```python
from build123d import *

# Parameters (mm, degrees)
F0_W     = 120
F0_H     = 60
F1_DEPTH = 3
F3_DEPTH = 1
F5_DEPTH = 1
F6_D     = 3.3
F7_D     = 3.3


with BuildPart() as f1:
    # F0 (on Top) → F1 (new body)
    with BuildSketch(Plane.XY):
        with Locations((63.9999989198, 30)):
            Rectangle(F0_W, F0_H)
    extrude(amount=F1_DEPTH)

    # F2 (on face) → F3 (cut)
    with BuildSketch(Plane.XY.offset(3)):
        with BuildLine():
            ThreePointArc((14.6999989198, 54.4), (13.2062435039, 58.0062445841), (9.5999989198, 59.5))
            Line((9.5999989198, 59.5), (9.5999989198, 54.4))
            Line((9.5999989198, 54.4), (14.6999989198, 54.4))
        make_face()
        with BuildLine():
            Line((9.5999989198, 49.3), (9.5999989198, 54.4))
            Line((9.5999989198, 54.4), (4.4999989198, 54.4))
            ThreePointArc((4.4999989198, 54.4), (5.9937543357, 50.7937554159), (9.5999989198, 49.3))
        make_face()
        with BuildLine():
            Line((14.6999989198, 54.4), (9.5999989198, 54.4))
            Line((9.5999989198, 54.4), (9.5999989198, 49.3))
            ThreePointArc((9.5999989198, 49.3), (13.2062435039, 50.7937554159), (14.6999989198, 54.4))
        make_face()
        with BuildLine():
            Line((9.5999989198, 5.6), (9.5999989198, 10.7))
            ThreePointArc((9.5999989198, 10.7), (5.9937543357, 9.2062445841), (4.4999989198, 5.6))
            Line((4.4999989198, 5.6), (9.5999989198, 5.6))
        make_face()
        with BuildLine():
            ThreePointArc((14.6999989198, 5.6), (13.2062435039, 9.2062445841), (9.5999989198, 10.7))
            Line((9.5999989198, 10.7), (9.5999989198, 5.6))
            Line((9.5999989198, 5.6), (14.6999989198, 5.6))
        make_face()
        with BuildLine():
            Line((9.5999989198, 5.6), (4.4999989198, 5.6))
            ThreePointArc((4.4999989198, 5.6), (5.9937543357, 1.9937554159), (9.5999989198, 0.5))
            Line((9.5999989198, 0.5), (9.5999989198, 5.6))
        make_face()
        with BuildLine():
            Line((14.6999989198, 5.6), (9.5999989198, 5.6))
            Line((9.5999989198, 5.6), (9.5999989198, 0.5))
            ThreePointArc((9.5999989198, 0.5), (13.2062435039, 1.9937554159), (14.6999989198, 5.6))
        make_face()
        with BuildLine():
            Line((118.3999989198, 5.6), (118.3999989198, 10.7))
            ThreePointArc((118.3999989198, 10.7), (114.7937543357, 9.2062445841), (113.2999989198, 5.6))
            Line((113.2999989198, 5.6), (118.3999989198, 5.6))
        make_face()
        with BuildLine():
            Line((118.3999989198, 5.6), (113.2999989198, 5.6))
            ThreePointArc((113.2999989198, 5.6), (114.7937543357, 1.9937554159), (118.3999989198, 0.5))
            Line((118.3999989198, 0.5), (118.3999989198, 5.6))
        make_face()
        with BuildLine():
            ThreePointArc((123.4999989198, 5.6), (122.0062435039, 9.2062445841), (118.3999989198, 10.7))
            Line((118.3999989198, 10.7), (118.3999989198, 5.6))
            Line((118.3999989198, 5.6), (123.4999989198, 5.6))
        make_face()
        with BuildLine():
            ThreePointArc((118.3999989198, 0.5), (122.0062435039, 1.9937554159), (123.4999989198, 5.6))
            Line((123.4999989198, 5.6), (118.3999989198, 5.6))
            Line((118.3999989198, 5.6), (118.3999989198, 0.5))
        make_face()
        with BuildLine():
            Line((118.3999989198, 54.4), (118.3999989198, 59.5))
            ThreePointArc((118.3999989198, 59.5), (114.7937543357, 58.0062445841), (113.2999989198, 54.4))
            Line((113.2999989198, 54.4), (118.3999989198, 54.4))
        make_face()
        with BuildLine():
            Line((118.3999989198, 54.4), (113.2999989198, 54.4))
            ThreePointArc((113.2999989198, 54.4), (114.7937543357, 50.7937554159), (118.3999989198, 49.3))
            Line((118.3999989198, 49.3), (118.3999989198, 54.4))
        make_face()
        with BuildLine():
            ThreePointArc((123.4999989198, 54.4), (122.0062435039, 58.0062445841), (118.3999989198, 59.5))
            Line((118.3999989198, 59.5), (118.3999989198, 54.4))
            Line((118.3999989198, 54.4), (123.4999989198, 54.4))
        make_face()
        with BuildLine():
            Line((123.4999989198, 54.4), (118.3999989198, 54.4))
            Line((118.3999989198, 54.4), (118.3999989198, 49.3))
            ThreePointArc((118.3999989198, 49.3), (122.0062435039, 50.7937554159), (123.4999989198, 54.4))
        make_face()
        with BuildLine():
            Line((9.5999989198, 54.4), (9.5999989198, 59.5))
            ThreePointArc((9.5999989198, 59.5), (5.9937543357, 58.0062445841), (4.4999989198, 54.4))
            Line((4.4999989198, 54.4), (9.5999989198, 54.4))
        make_face()
        with BuildLine():
            Line((9.5999989198, 59.5), (9.5999989198, 60))
            Line((9.5999989198, 60), (3.9999989198, 60))
            Line((3.9999989198, 60), (3.9999989198, 54.4))
            Line((3.9999989198, 54.4), (4.4999989198, 54.4))
            ThreePointArc((4.4999989198, 54.4), (5.9937543357, 58.0062445841), (9.5999989198, 59.5))
        make_face()
        with BuildLine():
            Line((123.9999989198, 60), (118.3999989198, 60))
            Line((118.3999989198, 60), (118.3999989198, 59.5))
            ThreePointArc((118.3999989198, 59.5), (122.0062435039, 58.0062445841), (123.4999989198, 54.4))
            Line((123.4999989198, 54.4), (123.9999989198, 54.4))
            Line((123.9999989198, 54.4), (123.9999989198, 60))
        make_face()
        with BuildLine():
            Line((123.9999989198, 0), (123.9999989198, 5.6))
            Line((123.9999989198, 5.6), (123.4999989198, 5.6))
            ThreePointArc((123.4999989198, 5.6), (122.0062435039, 1.9937554159), (118.3999989198, 0.5))
            Line((118.3999989198, 0.5), (118.3999989198, 0))
            Line((118.3999989198, 0), (123.9999989198, 0))
        make_face()
        with BuildLine():
            Line((4.4999989198, 5.6), (3.9999989198, 5.6))
            Line((3.9999989198, 5.6), (3.9999989198, 0))
            Line((3.9999989198, 0), (9.5999989198, 0))
            Line((9.5999989198, 0), (9.5999989198, 0.5))
            ThreePointArc((9.5999989198, 0.5), (5.9937543357, 1.9937554159), (4.4999989198, 5.6))
        make_face()
    extrude(amount=-F3_DEPTH, mode=Mode.SUBTRACT)

    # F4 (on face) → F5 (cut)
    with BuildSketch(Plane.XY.offset(3)):
        with BuildLine():
            add(Edge.make_bspline(
                [(63.9999989198, 60), (53.3078499409, 56.3984259531), (33.5495887668, 49.7075267127), (17.2264214287, 49.4590057291), (9.7372470228, 49.3018471033)],
                knots=[0, 0, 0, 0, 0.5410756029, 1, 1, 1, 1], degree=3))
            Line((63.9999989198, 60), (9.5999989198, 60))
            Line((9.5999989198, 60), (9.5999989198, 59.5))
            ThreePointArc((9.5999989198, 59.5), (14.6995371231, 54.4686302658), (9.7372470228, 49.3018471033))
        make_face()
        with BuildLine():
            Line((118.3999989198, 60), (63.9999989198, 60))
            add(Edge.make_bspline(
                [(63.9999989198, 60), (72.5641843861, 56.1127336818), (89.7555419494, 48.3096115422), (108.8285530179, 48.9690651334), (118.3999989198, 49.3)],
                knots=[0, 0, 0, 0, 0.4981680728, 1, 1, 1, 1], degree=3))
            ThreePointArc((118.3999989198, 49.3), (113.2999989198, 54.4), (118.3999989198, 59.5))
            Line((118.3999989198, 59.5), (118.3999989198, 60))
        make_face()
        with BuildLine():
            add(Edge.make_bspline(
                [(63.9999989198, 0), (72.1609270774, 2.9084131067), (88.7930843444, 8.835825192), (107.9878966542, 10.0624659865), (117.7781419332, 10.6619456623)],
                knots=[0, 0, 0, 0, 0.4854368856, 0.9893314178, 0.9893314178, 0.9893314178, 0.9893314178], degree=3))
            Line((63.9999989198, 0), (118.3999989198, 0))
            Line((118.3999989198, 0), (118.3999989198, 0.5))
            ThreePointArc((118.3999989198, 0.5), (113.3095213942, 5.28848987), (117.7781419332, 10.6619456623))
        make_face()
        with BuildLine():
            add(Edge.make_bspline(
                [(63.9999989198, 0), (55.110608048, 3.1316324942), (37.4637794456, 9.3648834823), (19.1775133134, 10.2247717324), (10.1042544322, 10.675009988)],
                knots=[0, 0, 0, 0, 0.5036943289, 1, 1, 1, 1], degree=3))
            ThreePointArc((10.1042544322, 10.675009988), (14.6937475855, 5.3475628185), (9.5999989198, 0.5))
            Line((9.5999989198, 0.5), (9.5999989198, 0))
            Line((9.5999989198, 0), (63.9999989198, 0))
        make_face()
    extrude(amount=-F5_DEPTH, mode=Mode.SUBTRACT)

    # F6 (through all)
    with Locations(Plane.XY.offset(3)):
        with Locations((9.5999989198, 54.4)):
            Hole(F6_D / 2)

    # F7 (through all)
    with Locations(Plane.XY.offset(3)):
        with Locations((118.3999989198, 54.4), (118.3999989198, 5.6), (9.5999989198, 5.6)):
            Hole(F7_D / 2)


solid = f1.part
```
Model file for the job. Use its own axes, mm. A direction names the side the tool comes from. Give positions to 0.01 mm unless a question says otherwise; leave off trailing zeros. One line per item, written item: value. Start each with the question number.
1. Which spindle directions (+Z, -Z, +X, -X, +Y, -Y) get a long thin tool onto all of the face, cutting with end or side? Do faces 5 (the flat face through (4, 30, 1)), 6 (the flat face through (27, 56, 2)), 7 (the flat face through (100, 4, 2)). Say none if no direction does.
2. Probe L1, parallel to Z at x = 38, y = 56; L2, parallel to Y at x = 89.5, z = 2.35; L3, parallel to Y at x = 18.5, z = 2.3. List the from-to ranges inside material, lowest first. Write a range as from..to.
3. Pin check, flat tips, straight feed: pin 1 (2 mm diameter, centred on x = 118.4, y = 54.4, fed in from +Z); pin 2 (3 mm diameter, centred on x = 29, y = 7.5, fed in from +Z). Stop position of each tip, or through.
4. Pull direction Y, two halves, no side cores. Call faces 1 (the cylindrical face through (116.876, 4.968, 0.986)), 2 (the cylindrical face through (117.639, 52.936, 0.986)), 3 (the flat face through (27, 4, 2)), 4 (the cylindrical face through (121.966, 50.754, 2.507)): pulls with the +Y half, pulls with the -Y half, needs draft (parallel to the pull), parting line crosses it, or undercut.
Solution:
1. face 5: +Z, -Z, -X, +Y, -Y
1. face 6: +Z, +Y
1. face 7: +Z, -Y
2. L1: z = 0..2
2. L2: y = 7.67..50.57
2. L3: y = 10.23..49.55
3. pin 1: passes through
3. pin 2: stops at z = 2
4. face 1: undercut
4. face 2: undercut
4. face 3: needs draft
4. face 4: pulls with the +Y half
